Can you work these out from the model? Positions are in its coordinate system, mm. Face numbers are marked on the shaded views. A direction names the side the tool comes from. Round coordinates to 2 decimals unless told otherwise and drop trailing zeros. Loops run counter-clockwise (first coordinate to the right, second up) from the corner with the lowest first, then second, coordinate; pieces in that order, holes last. Notation, with made-up numbers: M -29.5,88 L 27.5,88 A23 ccw 27.5,112 Z; hole C 75.5,45.25 d1. An arc over 180 degrees is marked long. Return JSON: item names as keys, results as strings.
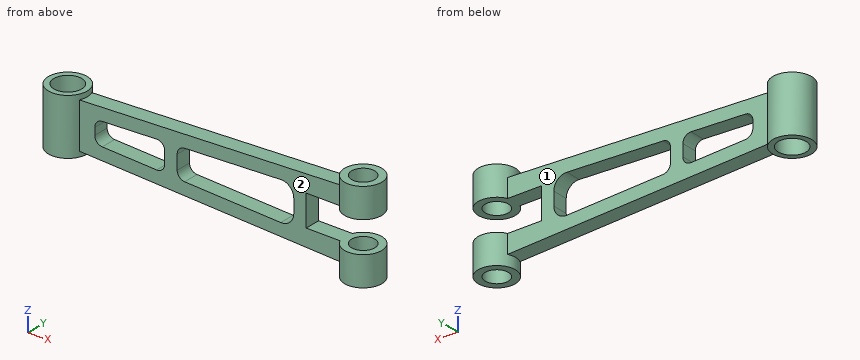
```python
from build123d import *

# Parameters (mm, degrees)
SKETCH1_R           = 12.5
BOSS_EXTRUDE1_DEPTH = 18
SKETCH2_R           = 12
BOSS_EXTRUDE2_DEPTH = 29
BOSS_EXTRUDE4_DEPTH = 5
SKETCH7_W           = 62.580609479
SKETCH7_H           = 20
CUT_EXTRUDE2_DEPTH  = 62
CUT_EXTRUDE3_DEPTH  = 62
SKETCH9_R           = 9
SKETCH9_R_2         = 7.5
CUT_EXTRUDE4_DEPTH  = 62


with BuildPart() as part:
    # Sketch1 → Boss-Extrude1 (new, symmetric)
    with BuildSketch(Plane.XY):
        with Locations((-95, 0)):
            Circle(SKETCH1_R)
    extrude(amount=BOSS_EXTRUDE1_DEPTH, both=True)



with BuildPart() as body_2:
    # Sketch2 → Boss-Extrude2 (new, symmetric)
    with BuildSketch(Plane.XY):
        with Locations(Location((95, 0, 0), (0, 0, 180))):
            Circle(SKETCH2_R)
    extrude(amount=BOSS_EXTRUDE2_DEPTH, both=True)


with BuildPart() as part_1:
    add(part.part)

    add(body_2.part)  # Boss-Extrude4 merges body 2
    # Sketch6 → Boss-Extrude4 (add, symmetric)
    with BuildSketch(Plane(origin=(0, 0, 0), x_dir=(1, 0, 0), z_dir=(0, 1, 0))):
        Polygon((95, 22.434972483), (95, -22.434972483), (-95, -14.13939333), (-95, 14.13939333), align=None)
    extrude(amount=BOSS_EXTRUDE4_DEPTH, both=True)

    # Sketch7 → Cut-Extrude2 (cut, symmetric)
    with BuildSketch(Plane(origin=(0, 5, 0), x_dir=(1, 0, 0), z_dir=(0, 1, 0))):
        with Locations((93.62091422, 0)):
            Rectangle(SKETCH7_W, SKETCH7_H)
    extrude(amount=CUT_EXTRUDE2_DEPTH, both=True, mode=Mode.SUBTRACT)

    # Sketch8 → Cut-Extrude3 (cut, symmetric)
    with BuildSketch(Plane(origin=(0, 5, 0), x_dir=(1, 0, 0), z_dir=(0, 1, 0))):
        with BuildLine():
            Line((-68.887487457, -7.271868768), (-33.887487457, -8.80000177))
            ThreePointArc((-33.887487457, -8.80000177), (-30.211825242, -7.416580473), (-28.66939052, -3.804760662))
            Line((-28.66939052, -3.804760662), (-28.66939052, 3.804760662))
            ThreePointArc((-28.66939052, 3.804760662), (-30.211825242, 7.416580473), (-33.887487457, 8.80000177))
            Line((-33.887487457, 8.80000177), (-68.887487457, 7.271868768))
            ThreePointArc((-68.887487457, 7.271868768), (-72.281210331, 5.734192939), (-73.66939052, 2.276627661))
            Line((-73.66939052, 2.276627661), (-73.66939052, -2.276627661))
            ThreePointArc((-73.66939052, -2.276627661), (-72.281210331, -5.734192939), (-68.887487457, -7.271868768))
        make_face()
        with BuildLine():
            Line((-20.66939052, 4.590657635), (-20.66939052, -4.590657635))
            ThreePointArc((-20.66939052, -4.590657635), (-19.281210331, -8.048222914), (-15.887487457, -9.585898743))
            Line((-15.887487457, -9.585898743), (45.981654381, -12.287163812))
            ThreePointArc((45.981654381, -12.287163812), (51.862713926, -10.073689736), (54.33060948, -4.29477804))
            Line((54.33060948, -4.29477804), (54.33060948, 4.29477804))
            ThreePointArc((54.33060948, 4.29477804), (51.862713926, 10.073689736), (45.981654381, 12.287163812))
            Line((45.981654381, 12.287163812), (-15.887487457, 9.585898743))
            ThreePointArc((-15.887487457, 9.585898743), (-19.281210331, 8.048222914), (-20.66939052, 4.590657635))
        make_face()
    extrude(amount=CUT_EXTRUDE3_DEPTH, both=True, mode=Mode.SUBTRACT)

    # Sketch9 → Cut-Extrude4 (cut, symmetric)
    with BuildSketch(Plane.XY):
        with Locations((-95, 0)):
            Circle(SKETCH9_R)
        with Locations((95, 0)):
            Circle(SKETCH9_R_2)
    extrude(amount=CUT_EXTRUDE4_DEPTH, both=True, mode=Mode.SUBTRACT)


solid = part_1.part
```
Q1. Suppose I cut it at D-D, the plane x = -2. Please give me the cut outline in (y, z), plus the area to 3 significant figures.
Results:
{"outline": "M -5,-18.2 L 5,-18.2 L 5,-10.19 L -5,-10.19 Z; M -5,10.19 L 5,10.19 L 5,18.2 L -5,18.2 Z", "area": "160 mm2"}
Q2. Suppose I cut it at C-C, the plane y = 0. State how many separate pieces and enclosed holes the cut face has, plus the area to 3 significant figures.
Results:
{"separate pieces": "4", "enclosed holes": "2", "area": "3,920 mm2"}
Q3. If I drill on line 1 along X through (y, z) = (-3.75, -13.5); line 2 along X through (y, z) = (3, -13); line 3 along Z through (x, y) = (91, 6.5), over which ranges is the centre line in solid material (lowest first)?
Results:
{"line 1": "x = -106.92 to -103.18, -86.82 to 88.5, 101.5 to 106.4", "line 2": "x = -107.13 to -103.49, -86.51 to 88.13, 101.87 to 106.62", "line 3": "z = -29 to -10, 10 to 29"}
Q4. I'm going to push flat-ended pins straight in: pin 1 Ø10 at (x, z) = (2, -13.5) entering from +Y; pin 2 Ø1 at (x, z) = (62.5, 13.5) entering from -Y; pin 3 Ø1 at (y, z) = (0.5, -8.5) entering from +X. Where does each tip first touch, or does it pass through?
Results:
{"pin 1": "stops at y = 5", "pin 2": "stops at y = -5", "pin 3": "stops at x = 62.33"}
Q5. Suppose I cut it at B-B, the plane x = -95. Please give me the cut outline in (y, z), plus the area to 3 significant figures.
Results:
{"outline": "M -12.5,-18 L -9,-18 L -9,18 L -12.5,18 Z; M 9,-18 L 12.5,-18 L 12.5,18 L 9,18 Z", "area": "252 mm2"}
Q6. On a 3-axis mill with a long thin cutter (end or side, diameter ignored), from which of +Z, -Z, +X, -X, +Y, -Y can I reach the whole of each face in a straight line? I mean the marked faces 1 and 2. Say none if no direction works.
Results:
{"face 1": "+Z, -Z, +Y", "face 2": "+Z, -Z, -Y"}
Q7. Suppose I cut it at A-A, the plane x = 95. Please give me the cut outline in (y, z), plus the area to 3 significant figures.
Results:
{"outline": "M -12,-29 L -7.5,-29 L -7.5,-10 L -12,-10 Z; M -12,10 L -7.5,10 L -7.5,29 L -12,29 Z; M 7.5,-29 L 12,-29 L 12,-10 L 7.5,-10 Z; M 7.5,10 L 12,10 L 12,29 L 7.5,29 Z", "area": "342 mm2"}
